```python
from build123d import *

# Parameters (mm, degrees)
BOSS_EXTRUDE1_DEPTH = 5
SKETCH2_R           = 3.25
SKETCH2_R_2         = 0.65
CUT_EXTRUDE1_DEPTH  = 5


with BuildPart() as part:
    # Sketch1 → Boss-Extrude1 (new body)
    with BuildSketch(Plane.XY):
        with BuildLine():
            ThreePointArc((0, -15), (15, 0), (0, 15))
            add(Edge.make_bspline(
                [(0, 15), (-14.230583968, 15.97401443), (-71.542634771, -23.896673221), (-95.29355487, -84.024349777)],
                knots=[0, 0, 0, 0, 1, 1, 1, 1], degree=3))
            ThreePointArc((-95.29355487, -84.024349777), (-89.29355487, -90.024349777), (-83.293554869, -84.024349777))
            add(Edge.make_bspline(
                [(0, -15), (-22.042025083, -17.979465659), (-40.938355496, -27.190384656), (-83.293554869, -84.024349777)],
                knots=[0, 0, 0, 0, 1, 1, 1, 1], degree=3))
        make_face()
    extrude(amount=BOSS_EXTRUDE1_DEPTH)

    # Sketch2 → Cut-Extrude1 (cut)
    with BuildSketch(Plane.XY.offset(5)):
        Circle(SKETCH2_R)
        with Locations((0, 7.25)):
            Circle(SKETCH2_R_2)
        with Locations((-7.25, 0)):
            Circle(SKETCH2_R_2)
        with Locations((0, -7.25)):
            Circle(SKETCH2_R_2)
        with Locations((7.25, 0)):
            Circle(SKETCH2_R_2)
    extrude(amount=-CUT_EXTRUDE1_DEPTH, mode=Mode.SUBTRACT)


solid = part.part
```
For this review, take the finished solid that the model builds, in its own axes (mm). Round coordinates to 2 decimals unless told otherwise and drop trailing zeros. Use a Markdown table: item, result.
Item 1: Draft analysis for pull direction X (two halves, no side actions). For faces 1 (the cylindrical face through (-2.579, -1.978, 2.535)), 2 (the cylindrical face through (15, 0, 2)), 3 (the flat face through (-40, -25, 0)), state which applies: +X half, -X half, draft (parallel to the pull), parting line (faces both ways), or undercut.
Resolved:
| item | result |
|---|---|
| face 1 | undercut |
| face 2 | +X half |
| face 3 | draft |
Item 2: For line 1 along Y through (x, z) = (7.25, 3.45); line 2 along Y through (x, z) = (3, 4); line 3 along X through (y, z) = (-84, 3.45), list the stretches that pass through material, from the lowest coordinate up. Write a range as [from, to].
Resolved:
| item | result |
|---|---|
| line 1 | y = [-13.13, -0.65], [0.65, 13.13] |
| line 2 | y = [-14.7, -1.25], [1.25, 14.7] |
| line 3 | x = [-95.28, -83.28] |
Item 3: For pin 1 (2 mm diameter, centred on y = -7, z = 1.5, fed in from +X); pin 2 (2 mm diameter, centred on x = -43, z = 3.5, fed in from +Y); pin 3 (3 mm diameter, centred on y = -55.5, z = 2, fed in from +X), all flat-tipped, find the tip position at first contact; note any pin that passes through.
Resolved:
| item | result |
|---|---|
| pin 1 | stops at x = 13.75 |
| pin 2 | stops at y = -9.73 |
| pin 3 | stops at x = -59.35 |
Item 4: Take a section at A-A (z = 2.05). State how many separate pieces and enclosed holes the cut face has, plus the area to 3 significant figures.
Resolved:
| item | result |
|---|---|
| separate pieces | 1 |
| enclosed holes | 5 |
| area | 2,790 mm² |
